For this review, take the finished solid that the model builds, in its own axes (mm). Round coordinates to 2 decimals unless told otherwise and drop trailing zeros. Order: outer loops, then holes, each group sorted by start corner. A loop starts at its lowest first (then second) coordinate and runs counter-clockwise, first axis right, second up. Notation, with made-up numbers: (54, 32.5) - (106, 32.5) arc R30 cw to (106, 66.5) - close; hole circle Ø6 at (-39.75, 18). An arc over 180 degrees is marked (long way). One line per question, with ' | ' between items.
```python
from build123d import *

# Parameters (mm, degrees)
F_1_4_20_TAPPED_HOLE1_D           = 5.1054
F_1_4_20_TAPPED_HOLE1_DEPTH       = 76.2
F_1_4_20_TAPPED_HOLE1_CSINK_D     = 7.62
F_1_4_20_TAPPED_HOLE1_CSINK_ANGLE = 100
F_1_4_0_25_DIAMETER_HOLE1_D       = 6.35


with BuildPart() as part:
    # Sketch1 → Revolve1 (revolve)
    with BuildSketch(Plane(origin=(0, 0, 0), x_dir=(-1, 0, 0), z_dir=(0, 0, -1))):
        Polygon((-5.83819, 0), (0, 0), (0, 76.2), (-5.83819, 76.2), (-6.34619, 75.692), (-6.34619, 0.508), align=None)
    revolve(axis=Axis((0, 0, 0), (0, 1, 0)))

    # 1/4-20 Tapped Hole1
    with Locations(Plane(origin=(0, 76.2, 0), x_dir=(1, 0, 0), z_dir=(0, 1, 0))):
        with Locations((0, 0)):
            CounterSinkHole(F_1_4_20_TAPPED_HOLE1_D / 2, F_1_4_20_TAPPED_HOLE1_CSINK_D / 2, depth=F_1_4_20_TAPPED_HOLE1_DEPTH, counter_sink_angle=F_1_4_20_TAPPED_HOLE1_CSINK_ANGLE)

    # 1/4 (0.25) Diameter Hole1 (through all)
    with Locations(Plane(origin=(-5.114677075, 17.430811078, -3.756887799), x_dir=(0.591991068, 0, -0.805944523), z_dir=(-0.805944523, 0, -0.591991068))):
        with Locations((0, 0)):
            Hole(F_1_4_0_25_DIAMETER_HOLE1_D / 2)


solid = part.part
```
(1) We need section A-A on z = 1.75. Give the number of separate pieces and of enclosed holes in the cut face, plus the area to 3 significant figures.
Output values:
separate pieces: 3 | enclosed holes: 0 | area: 616 mm^2
(2) Insertion check: pin 1 (4 mm diameter, centred on y = 61.5, z = -0.5, fed in from -X); pin 2 (3 mm diameter, centred on y = 62, z = -2.5, fed in from +X); pin 3 (5 mm diameter, centred on x = 0, z = 1, fed in from +Y). Each pin has a flat end and moves straight along its axis. Give the tip position at first contact, or say it passes through.
Output values:
pin 1: x = -6.35 | pin 2: x = 6.27 | pin 3: y = 75.94
(3) We need section B-B on y = 29. State the section outline as (x, z) points, plus the area to 3 significant figures.
Output values:
outline: circle Ø12.69 at (0, 0); hole circle Ø5.11 at (0, 0) | area: 106 mm^2
(4) For probe 1 along Z at (x, y) = (0, 11.5); probe 2 along Y at (x, z) = (-4.25, 0); probe 3 along X at (y, z) = (26, 0.5), list the stretches that pass through material, from the lowest coordinate up. Write a range as [from, to].
Output values:
probe 1: [-6.35, -2.55], [2.55, 6.35] | probe 2: [0, 15.49], [19.37, 76.2] | probe 3: [-6.33, -2.5], [2.5, 6.33]
(5) Mouldability with a two-part tool opening along X and no side actions: class faces 1 (the cylindrical face through (-2.435, 46.841, -0.767)), 2 (the flat face through (3, 0, 1)), 3 (the cylindrical face through (3.41, 37.57, -5.35)) as released by +X, released by -X, zero draft, split by the parting line, or undercut.
Output values:
face 1: undercut | face 2: zero draft | face 3: split by the parting line
